from build123d import *

# Parameters (mm, degrees)
SKETCH_1_R               = 23.5
SKETCH_1_R_2             = 1.5
EXTRUDE_1_DEPTH          = 10
SKETCH_2_R               = 28.5
SKETCH_2_R_2             = 23.5
EXTRUDE_2_DEPTH          = 25
SKETCH_5_W               = 55
SKETCH_5_H               = 10
CUT_EXTRUDE_1_DEPTH      = 9
RIB_6_REACH              = 55.364
SKETCH_7_WALL_W          = 123.679532162
SKETCH_7_WALL_H          = 10
CUT_EXTRUDE_2_DEPTH      = 1
CUT_EXTRUDE_2_DEPTH_BACK = 3
CUT_EXTRUDE_2_START      = 10
EXTRUDE_START            = -3.7
EXTRUDE_3_DEPTH          = 2.7
EXTRUDE_START_2          = -6.7
EXTRUDE_5_DEPTH          = 3


with BuildPart() as part:
    # 草图1 → 凸台-拉伸1 (new body)
    with BuildSketch(Plane(origin=(0, 0, 0), x_dir=(1, 0, 0), z_dir=(0, 1, 0))):
        Polygon((-23.015398282, 33.05), (23.015398282, 33.05), (33.622, 22.443398282), (33.622, -22.443398282), (23.015398282, -33.05), (-23.015398282, -33.05), (-33.622, -22.443398282), (-33.622, 22.443398282), align=None)
        with Locations(Location((0, 0, 0), (0, 0, 270))):
            Circle(SKETCH_1_R, mode=Mode.SUBTRACT)
        with Locations(Location((-23.622, 18.669, 0), (0, 0, 270))):
            Circle(SKETCH_1_R_2, mode=Mode.SUBTRACT)
        with Locations(Location((23.622, 18.669, 0), (0, 0, 270))):
            Circle(SKETCH_1_R_2, mode=Mode.SUBTRACT)
        with Locations(Location((23.622, -18.669, 0), (0, 0, 270))):
            Circle(SKETCH_1_R_2, mode=Mode.SUBTRACT)
        with Locations(Location((-23.622, -18.669, 0), (0, 0, 270))):
            Circle(SKETCH_1_R_2, mode=Mode.SUBTRACT)
    extrude(amount=EXTRUDE_1_DEPTH)

    # 草图2 → 凸台-拉伸2 (add)
    with BuildSketch(Plane(origin=(0, 0, 0), x_dir=(1, 0, 0), z_dir=(0, 1, 0))):
        with Locations(Location((0, 0, 0), (0, 0, 90))):
            Circle(SKETCH_2_R)
        with Locations(Location((0, 0, 0), (0, 0, 270))):
            Circle(SKETCH_2_R_2, mode=Mode.SUBTRACT)
    extrude(amount=EXTRUDE_2_DEPTH)

    # 草图5 → 切除-拉伸1 (cut)
    with BuildSketch(Plane(origin=(0, 0, 0), x_dir=(1, 0, 0), z_dir=(0, 1, 0))):
        Rectangle(SKETCH_5_W, SKETCH_5_H)
    extrude(amount=CUT_EXTRUDE_1_DEPTH, mode=Mode.SUBTRACT)

    # 草图7 wall → 筋6 (add, up to next)
    with BuildSketch(Plane(origin=(-28.336, 15.286, 0), x_dir=(0.707106781187, 0.707106781187, 0), z_dir=(-0.707106781187, 0.707106781187, 0)), mode=Mode.PRIVATE) as rib_6_sk1:
        Rectangle(SKETCH_7_WALL_W, SKETCH_7_WALL_H)
    rib_6_tool1 = extrude(rib_6_sk1.sketch, amount=-RIB_6_REACH, mode=Mode.PRIVATE) - part.part
    rib_6 = rib_6_tool1.solids().sort_by_distance((-28.336, 15.286, 0))[0]
    add(rib_6)

    # 镜向1: 筋6 across plane
    add(rib_6.mirror(Plane(origin=(0, 0, 0), x_dir=(0, 0, 1), z_dir=(1, 0, 0))))

    # 草图9 → 切除-拉伸2 (cut, two sides: drawn at the far end of the back side and taken through both)
    with BuildSketch(Plane(origin=(0, 0, 0), x_dir=(1, 0, 0), z_dir=(0, 1, 0)).offset(CUT_EXTRUDE_2_START - CUT_EXTRUDE_2_DEPTH_BACK)):
        Polygon((-24.807031722, -21.615019883), (-21.663187802, -21.168277517), (-20.47815608, -18.222257634), (-22.436968278, -15.722980117), (-25.580812198, -16.169722483), (-26.76584392, -19.115742366), align=None)
        Polygon((26.76584392, -19.115742366), (25.580812198, -16.169722483), (22.436968278, -15.722980117), (20.47815608, -18.222257634), (21.663187802, -21.168277517), (24.807031722, -21.615019883), align=None)
        Polygon((25.601030295, 16.185701302), (26.762114905, 19.141241161), (24.783084611, 21.624539859), (21.642969705, 21.152298698), (20.481885095, 18.196758839), (22.460915389, 15.713460141), align=None)
        Polygon((-25.601030295, 16.185701302), (-22.460915389, 15.713460141), (-20.481885095, 18.196758839), (-21.642969705, 21.152298698), (-24.783084611, 21.624539859), (-26.762114905, 19.141241161), align=None)
    extrude(amount=CUT_EXTRUDE_2_DEPTH + CUT_EXTRUDE_2_DEPTH_BACK, mode=Mode.SUBTRACT)

    # 草图10 → 凸台-拉伸3 (add)
    with BuildSketch(Plane(origin=(0, 25, 0), x_dir=(1, 0, 0), z_dir=(0, 1, 0)).offset(EXTRUDE_START)):
        with BuildLine():
            ThreePointArc((-6.121524921, 22.688696142), (-12.673279961, 19.78984525), (-18.047118042, 15.051628828))
            Line((-18.047118042, 15.051628828), (-16.70318372, 13.930762851))
            ThreePointArc((-16.70318372, 13.930762851), (-11.72952507, 18.31613337), (-5.665666682, 20.999112387))
            Line((-5.665666682, 20.999112387), (-6.121524921, 22.688696142))
        make_face()
        with BuildLine():
            Line((-3.712802663, 21.430762851), (-4.011533912, 23.155077104))
            ThreePointArc((-4.011533912, 23.155077104), (-5.071892953, 22.946152224), (-6.121524921, 22.688696142))
            Line((-6.121524921, 22.688696142), (-5.665666682, 20.999112387))
            ThreePointArc((-5.665666682, 20.999112387), (-4.694198797, 21.237396207), (-3.712802663, 21.430762851))
        make_face()
        with BuildLine():
            Line((21.018598125, -5.592944917), (22.709749699, -6.04295198))
            ThreePointArc((22.709749699, -6.04295198), (23.301599923, -3.047202166), (23.5, 0))
            ThreePointArc((23.5, 0), (23.136857186, 4.115317671), (22.058651954, 8.103448276))
            Line((22.058651954, 8.103448276), (20.415986383, 7.5))
            ThreePointArc((20.415986383, 7.5), (21.413899736, 3.808857845), (21.75, 0))
            ThreePointArc((21.75, 0), (21.566374397, -2.820282856), (21.018598125, -5.592944917))
        make_face()
        with BuildLine():
            Line((20.415986383, -7.5), (22.058651954, -8.103448276))
            ThreePointArc((22.058651954, -8.103448276), (22.407897221, -7.080687969), (22.709749699, -6.04295198))
            Line((22.709749699, -6.04295198), (21.018598125, -5.592944917))
            ThreePointArc((21.018598125, -5.592944917), (20.739224024, -6.553402695), (20.415986383, -7.5))
        make_face()
        with BuildLine():
            ThreePointArc((-16.588224778, -16.645744163), (-10.801868743, -20.870305021), (-4.011533912, -23.155077104))
            Line((-4.011533912, -23.155077104), (-3.712802663, -21.430762851))
            ThreePointArc((-3.712802663, -21.430762851), (-9.997474263, -19.31613337), (-15.352931443, -15.40616747))
            Line((-15.352931443, -15.40616747), (-16.588224778, -16.645744163))
        make_face()
        with BuildLine():
            ThreePointArc((-18.047118042, -15.051628828), (-17.336004268, -15.865464255), (-16.588224778, -16.645744163))
            Line((-16.588224778, -16.645744163), (-15.352931443, -15.40616747))
            ThreePointArc((-15.352931443, -15.40616747), (-16.045025227, -14.683993512), (-16.70318372, -13.930762851))
            Line((-16.70318372, -13.930762851), (-18.047118042, -15.051628828))
        make_face()
    extrude(amount=EXTRUDE_3_DEPTH)

    # 草图10<3> → 凸台-拉伸5 (add)
    with BuildSketch(Plane(origin=(0, 25, 0), x_dir=(1, 0, 0), z_dir=(0, 1, 0)).offset(EXTRUDE_START_2)):
        with BuildLine():
            Line((-3.712802663, 21.430762851), (-4.011533912, 23.155077104))
            ThreePointArc((-4.011533912, 23.155077104), (-5.071892953, 22.946152224), (-6.121524921, 22.688696142))
            Line((-6.121524921, 22.688696142), (-5.665666682, 20.999112387))
            ThreePointArc((-5.665666682, 20.999112387), (-4.694198797, 21.237396207), (-3.712802663, 21.430762851))
        make_face()
        with BuildLine():
            ThreePointArc((-18.047118042, -15.051628828), (-17.336004268, -15.865464255), (-16.588224778, -16.645744163))
            Line((-16.588224778, -16.645744163), (-15.352931443, -15.40616747))
            ThreePointArc((-15.352931443, -15.40616747), (-16.045025227, -14.683993512), (-16.70318372, -13.930762851))
            Line((-16.70318372, -13.930762851), (-18.047118042, -15.051628828))
        make_face()
        with BuildLine():
            Line((20.415986383, -7.5), (22.058651954, -8.103448276))
            ThreePointArc((22.058651954, -8.103448276), (22.407897221, -7.080687969), (22.709749699, -6.04295198))
            Line((22.709749699, -6.04295198), (21.018598125, -5.592944917))
            ThreePointArc((21.018598125, -5.592944917), (20.739224024, -6.553402695), (20.415986383, -7.5))
        make_face()
    extrude(amount=EXTRUDE_5_DEPTH)


solid = part.part
Input: part model. Units: mm. Frame: model coordinates. A direction names the side the tool comes from. Round coordinates to 2 decimals unless told otherwise and drop trailing zeros. Loops run counter-clockwise (first coordinate to the right, second up) from the corner with the lowest first, then second, coordinate; pieces in that order, holes last. Notation, with made-up numbers: (35, 57.25) -> (77, 57.25) arc R11 ccw to (77, 67.25) -> close; hole circle Ø5 at (80.5, 41.5). An arc over 180 degrees is marked (long way). Answer as a JSON object with one key per item and string values. Group by question number.
1) Reachability of faces 1 (the flat face through (-25.8, 8.48, 20.35)), 2 (the flat face through (21.249, 22.631, -7.806)), 3 (the flat face through (-21.485, 8.972, -16.938)), 4 (the flat face through (-25, 9, 0)) from +Z, -Z, +X, -X, +Y, -Y: full face, straight path, thin tool, end or side. Return the list, or none.
2) Pin query (flat end, axial travel): pin 1 (1.1 mm diameter, centred on x = 21.5, z = 6.5, fed in from -Y); pin 2 (2.5 mm diameter, centred on x = 26.5, y = 4, fed in from -Z); pin 3 (1 mm diameter, centred on x = 8.5, y = 20, fed in from +Z); pin 4 (12 mm diameter, centred on x = 12, z = -0.5, fed in from +Y). Return the tip coordinate at first contact, or that it passes through.
3) Section query D-D on y = 2. Output: boundary loops of the cut face in (x, z), plus the area to 3 significant figures.
4) Section query A-A on x = 0. Output: boundary loops of the cut face in (y, z).
5) Section query C-C on x = -19.5. Output: boundary loops of the cut face in (y, z), plus the area to 3 significant figures.
6) Draft query along X for faces 5 (the cylindrical face through (-22.941, 12.325, -5.094)), 6 (the flat face through (-12, 21.3, -19)), 7 (the flat face through (-30, 12, 5)), 8 (the flat face through (-28.244, 4.93, 27.821)). Return one class per face: +X half, -X half, draft (parallel to the pull), parting line (faces both ways), or undercut.
7) Ray query, L1, parallel to X at y = 5.5, z = -4; L2, parallel to X at y = 13, z = -8; L3, parallel to Z at x = 20, y = 13.5. Return the intervals inside material, ascending.
8) Section query B-B on y = 19.25. Output: boundary loops of the cut face in (x, z).
Reply:
{
 "1": {"face 1": "+Y", "face 2": "+Y, -Y", "face 3": "none", "face 4": "-Y"},
 "2": {"pin 1": "stops at y = 18.3", "pin 2": "stops at z = -30.82", "pin 3": "stops at z = 27.35", "pin 4": "passes through"},
 "3": {"outline": "(-33.62, -22.44) -> (-23.02, -33.05) -> (23.02, -33.05) -> (33.62, -22.44) -> (33.62, 22.44) -> (23.02, 33.05) -> (-23.02, 33.05) -> (-33.62, 22.44) -> close; hole (-27.5, -5) -> (-22.96, -5) arc R23.5 ccw to (22.96, -5) -> (27.5, -5) -> (27.5, 5) -> (22.96, 5) arc R23.5 ccw to (-22.96, 5) -> (-27.5, 5) -> close; hole circle Ø3 at (-23.62, -18.67); hole circle Ø3 at (-23.62, 18.67); hole circle Ø3 at (23.62, -18.67); hole circle Ø3 at (23.62, 18.67)", "area": "2,370 mm2"},
 "4": {"outline": "(0, -33.05) -> (10, -33.05) -> (10, -28.5) -> (25, -28.5) -> (25, -23.5) -> (0, -23.5) -> close; (0, 23.5) -> (25, 23.5) -> (25, 28.5) -> (10, 28.5) -> (10, 33.05) -> (0, 33.05) -> close"},
 "5": {"outline": "(0, -33.05) -> (10, -33.05) -> (10, -20.78) -> (25, -20.78) -> (25, -13.11) -> (0, -13.11) -> close; (0, 13.11) -> (25, 13.11) -> (25, 20.78) -> (10, 20.78) -> (10, 33.05) -> (0, 33.05) -> close", "area": "629 mm2"},
 "6": {"face 5": "undercut", "face 6": "undercut", "face 7": "draft", "face 8": "-X half"},
 "7": {"L1": "x = -33.62 to -27.5, 27.5 to 33.62", "L2": "x = -27.35 to -22.1, 22.1 to 27.35", "L3": "z = -20.3 to -12.34, 12.34 to 20.3"},
 "8": {"outline": "circle Ø57 at (0, 0); hole (-18.05, 15.05) arc R23.5 ccw to (-6.12, -22.69) -> (-5.67, -21) arc R21.75 ccw to (-3.71, -21.43) -> (-4.01, -23.16) arc R23.5 ccw to (22.71, 6.04) -> (21.02, 5.59) arc R21.75 ccw to (20.42, 7.5) -> (22.06, 8.1) arc R23.5 ccw to (-16.59, 16.65) -> (-15.35, 15.41) arc R21.75 ccw to (-16.7, 13.93) -> close"}
}
